```python
from build123d import *

# Parameters (mm, degrees)
SKETCH1_R           = 2
BOSS_EXTRUDE1_DEPTH = 3.175


with BuildPart() as part:
    # Sketch1 → Boss-Extrude1 (new body)
    with BuildSketch(Plane.XY):
        with BuildLine():
            Line((-40.75, 0), (40.75, 0))
            ThreePointArc((40.75, 0), (42.164213562, -0.585786438), (42.75, -2))
            Line((42.75, -2), (42.75, -97.5))
            ThreePointArc((42.75, -97.5), (42.164213562, -98.914213562), (40.75, -99.5))
            Line((40.75, -99.5), (-40.75, -99.5))
            ThreePointArc((-40.75, -99.5), (-42.164213562, -98.914213562), (-42.75, -97.5))
            Line((-42.75, -97.5), (-42.75, -2))
            ThreePointArc((-42.75, -2), (-42.164213562, -0.585786438), (-40.75, 0))
        make_face()
        with Locations((35, -89.975)):
            Circle(SKETCH1_R, mode=Mode.SUBTRACT)
        with Locations((-35, -89.975)):
            Circle(SKETCH1_R, mode=Mode.SUBTRACT)
        with Locations((35, -70.925)):
            Circle(SKETCH1_R, mode=Mode.SUBTRACT)
        with Locations((35, -28.58)):
            Circle(SKETCH1_R, mode=Mode.SUBTRACT)
        with Locations((-35, -70.92)):
            Circle(SKETCH1_R, mode=Mode.SUBTRACT)
        with Locations((-35, -28.58)):
            Circle(SKETCH1_R, mode=Mode.SUBTRACT)
    extrude(amount=BOSS_EXTRUDE1_DEPTH)


solid = part.part
```
For this review, take the finished solid that the model builds, in its own axes (mm). Round coordinates to 2 decimals unless told otherwise and drop trailing zeros. Order: outer loops, then holes, each group sorted by start corner. A loop starts at its lowest first (then second) coordinate and runs counter-clockwise, first axis right, second up.
Q1. Wall thickness on line 1 (Y direction, x = -35, z = 2.05) (3 decimals); line 2 (X direction, y = -90.5, z = 2.3): over which ranges is each line inside the solid? List them lowest first.
Findings below:
line 1: y = -99.5 to -91.975, -87.975 to -72.92, -68.92 to -30.58, -26.58 to 0
line 2: x = -42.75 to -36.93, -33.07 to 33.07, 36.93 to 42.75
Q2. We need section A-A, the plane x = 35. Give the boundary of the cut face in (y, z) (3 decimals), plus the area to 3 significant figures.
Findings below:
outline: (-99.5, 0) - (-91.975, 0) - (-91.975, 3.175) - (-99.5, 3.175) - close; (-87.975, 0) - (-72.925, 0) - (-72.925, 3.175) - (-87.975, 3.175) - close; (-68.925, 0) - (-30.58, 0) - (-30.58, 3.175) - (-68.925, 3.175) - close; (-26.58, 0) - (0, 0) - (0, 3.175) - (-26.58, 3.175) - close
area: 278 mm2
Q3. We need section B-B, the plane y = -28.58. Give the boundary of the cut face in (x, z) (3 decimals), plus the area to 3 significant figures.
Findings below:
outline: (-42.75, 0) - (-37, 0) - (-37, 3.175) - (-42.75, 3.175) - close; (-33, 0) - (33, 0) - (33, 3.175) - (-33, 3.175) - close; (37, 0) - (42.75, 0) - (42.75, 3.175) - (37, 3.175) - close
area: 246 mm2
Q4. Mouldability with a two-part tool opening along X and no side actions: class faces 1 (the cylindrical face through (-42.18, -0.6, 1.57)), 2 (the cylindrical face through (34.74, -68.94, 1.57)), 3 (the flat face through (1, -49, 3.175)) as pulls with the +X half, pulls with the -X half, needs draft (parallel to the pull), parting line crosses it, or undercut.
Findings below:
face 1: pulls with the -X half
face 2: undercut
face 3: needs draft
Q5. Insertion check: P1, Ø6.5, axis at x = 35, y = -28.58, coming from the -Z side; P2, Ø3.5, axis at x = 35, y = -89.975, coming from the -Z side. Each pin has a flat end and moves straight along its axis. Give the tip position at first contact, or say it passes through.
Findings below:
P1: stops at z = 0
P2: passes through
